Answer from the drawing. Dimensions are ordinates in mm from the lowest x, y and z of the part. A direction names the side the tool comes from. Give positions to 0.01 mm unless a question says otherwise; leave off trailing zeros. Order: outer loops, then holes, each group sorted by start corner. A loop starts at its lowest first (then second) coordinate and runs counter-clockwise, first axis right, second up. Notation, with made-up numbers: (61, -2.5) -> (77, -2.5) arc R22 ccw to (77, 32.5) -> close; hole circle Ø9 at (9, 87.25). An arc over 180 degrees is marked (long way). Answer as CSV lines item,"result". Start each with the question number.
1) Straight lines are drawn through the part: L1, parallel to Z at x = 4, y = 18; L2, parallel to X at y = 18, z = 3; L3, parallel to Y at x = 2.5, z = 1.75. For each, find the intervals that lie inside material, in ascending order. Write a range as from..to.
2) Find section A-A (y = 3). Determine the outline of the cut face in (x, z).
3) For the marked faces 4 and 5, determine the directions among +Z, -Z, +X, -X, +Y, -Y from which every point of the face is accessible in a straight line to the end or side of a thin tool.
4) Find section B-B (z = 3). Determine the outline of the cut face in (x, y), and give its area (3 significant figures).
5) The mould has two halves that part along X. Classify the marked faces 1, 2 and 3: +X half, -X half, draft (parallel to the pull), parting line (faces both ways), or undercut.
6) Find section D-D (z = 26). Determine the outline of the cut face in (x, y).
7) Flat-ended cylindrical pins translate along their axes: pin 1 Ø1 at (x, y) = (1.5, 3) entering from -Z; pin 2 Ø4.5 at (x, z) = (4, 3) entering from +Y. Find the tip coordinate at first contact, or state that the pin passes through.
8) Find section C-C (x = 4). Determine the outline of the cut face in (y, z), and give its area (3 significant figures).
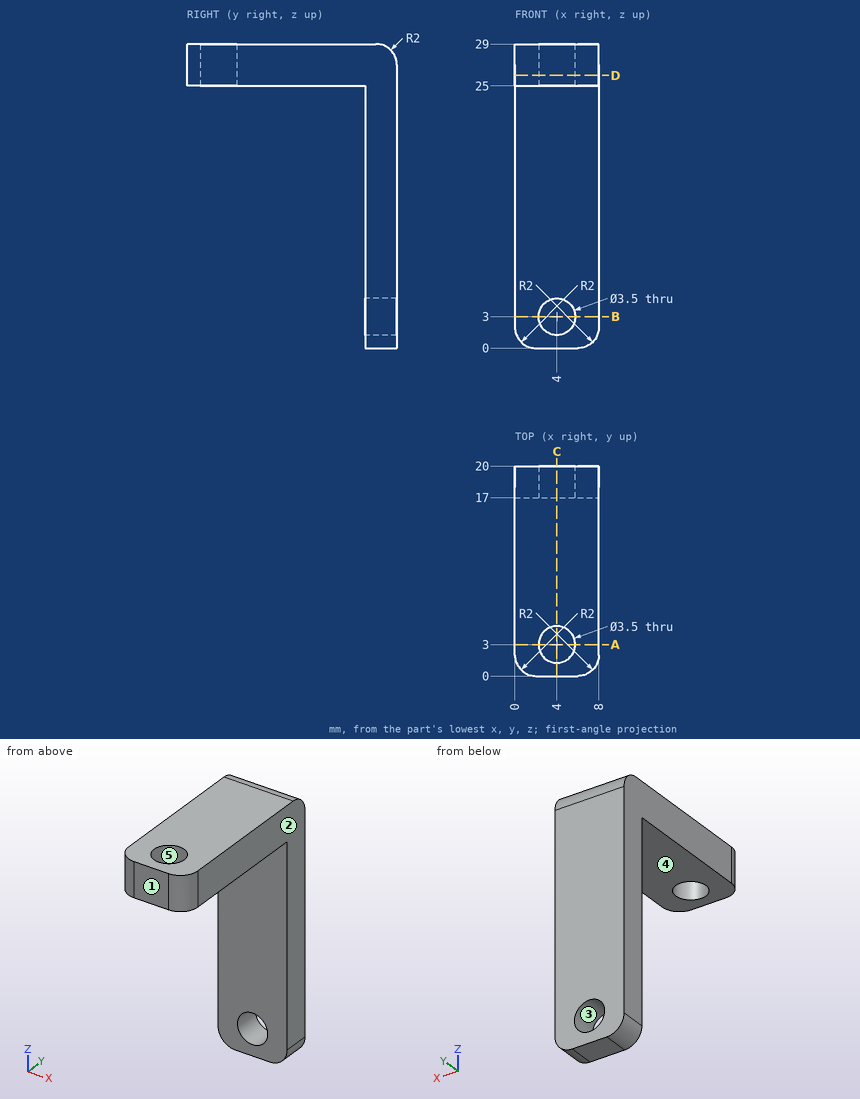
Findings below:
1,L1,"0..1.25, 4.75..29"
1,L2,"0..2.25, 5.75..8"
1,L3,"17..20"
2,outline,"(0, 25) -> (2.25, 25) -> (2.25, 29) -> (0, 29) -> close; (5.75, 25) -> (8, 25) -> (8, 29) -> (5.75, 29) -> close"
3,face 4,"-Z, +X, -X, -Y"
3,face 5,"+Z, -Z"
4,outline,"(0, 17) -> (2.25, 17) -> (2.25, 20) -> (0, 20) -> close; (5.75, 17) -> (8, 17) -> (8, 20) -> (5.75, 20) -> close"
4,area,"13.5 mm²"
5,face 1,"draft"
5,face 2,"+X half"
5,face 3,"undercut"
6,outline,"(0, 2) arc R2 ccw to (2, 0) -> (6, 0) arc R2 ccw to (8, 2) -> (8, 20) -> (0, 20) -> close; hole circle Ø3.5 at (4, 3)"
7,pin 1,"z = 25"
7,pin 2,"y = 20"
8,outline,"(0, 25) -> (1.25, 25) -> (1.25, 29) -> (0, 29) -> close; (4.75, 25) -> (17, 25) -> (17, 4.75) -> (20, 4.75) -> (20, 27) arc R2 ccw to (18, 29) -> (4.75, 29) -> close; (17, 0) -> (20, 0) -> (20, 1.25) -> (17, 1.25) -> close"
8,area,"130 mm²"
